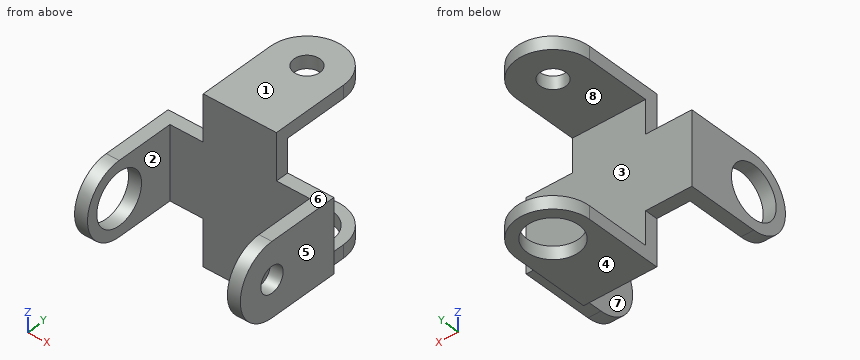
from build123d import *

# Parameters (mm, degrees)
BOSS_EXTRUDE1_DEPTH  = 5
SKETCH2_R            = 2.05
CUT_EXTRUDE1_DEPTH   = 5
SKETCH3_W            = 28.284271247
SKETCH3_H            = 5
BOSS_EXTRUDE3_DEPTH  = 5
SKETCH4_W            = 28.284271247
SKETCH4_H            = 5
BOSS_EXTRUDE4_DEPTH  = 54.01
BOSS_EXTRUDE5_DEPTH  = 5
SKETCH6_W            = 14.142135624
SKETCH6_H            = 14.14215
SKETCH6_W_2          = 12.862864377
SKETCH6_W_3          = 14.142135623
SKETCH6_W_4          = 12.862864376
BOSS_EXTRUDE7_DEPTH  = 5
SKETCH8_W            = 28.2843
SKETCH8_H            = 5
BOSS_EXTRUDE8_DEPTH  = 5
SKETCH10_W           = 5
SKETCH10_H           = 28.2843
BOSS_EXTRUDE9_DEPTH  = 22.6808
BOSS_EXTRUDE10_DEPTH = 5
SKETCH12_W           = 28.2843
SKETCH12_H           = 5
BOSS_EXTRUDE11_DEPTH = 5
BOSS_EXTRUDE12_START = -5
BOSS_EXTRUDE12_DEPTH = 5
SKETCH15_R           = 5
CUT_EXTRUDE3_DEPTH   = 5
SKETCH16_R           = 5
CUT_EXTRUDE4_DEPTH   = 14.1
SKETCH17_R           = 2.05
CUT_EXTRUDE5_DEPTH   = 8.1
SKETCH18_R           = 10
CUT_EXTRUDE6_DEPTH   = 5
SKETCH19_R           = 10
CUT_EXTRUDE7_DEPTH   = 5


with BuildPart() as part:
    # Model → Boss-Extrude1 (new body)
    with BuildSketch(Plane.XY):
        with BuildLine():
            Line((13.86155204, 4.132702322), (42.145823287, 4.132702322))
            Line((42.145823287, 4.132702322), (42.145823287, 29.132702322))
            ThreePointArc((42.145823287, 29.132702322), (28.003687664, 43.274837946), (13.86155204, 29.132702322))
            Line((13.86155204, 29.132702322), (13.86155204, 4.132702322))
        make_face()
    extrude(amount=BOSS_EXTRUDE1_DEPTH)

    # Sketch2 → Cut-Extrude1 (cut)
    with BuildSketch(Plane.XY.offset(5)):
        with Locations((28.003687664, 29.132702322)):
            Circle(SKETCH2_R)
    extrude(amount=-CUT_EXTRUDE1_DEPTH, mode=Mode.SUBTRACT)

    # Sketch3 → Boss-Extrude3 (add)
    with BuildSketch(Plane.XZ.offset(-4.132702322)):
        with Locations((28.003687664, 2.5)):
            Rectangle(SKETCH3_W, SKETCH3_H)
    extrude(amount=BOSS_EXTRUDE3_DEPTH)

    # Sketch4 → Boss-Extrude4 (add)
    with BuildSketch(Plane.XY.offset(5)):
        with Locations((28.003687664, 1.632702322)):
            Rectangle(SKETCH4_W, SKETCH4_H)
    extrude(amount=BOSS_EXTRUDE4_DEPTH)

    # Sketch5 → Boss-Extrude5 (add)
    with BuildSketch(Plane.XY.offset(59.01)):
        with BuildLine():
            Line((42.145823287, 4.132702322), (42.145823287, 29.132702322))
            ThreePointArc((42.145823287, 29.132702322), (28.003687664, 43.274837946), (13.86155204, 29.132702322))
            Line((13.86155204, 29.132702322), (13.86155204, 4.132702322))
            Line((13.86155204, 4.132702322), (13.86155204, -0.867297678))
            Line((13.86155204, -0.867297678), (42.145823287, -0.867297678))
            Line((42.145823287, -0.867297678), (42.145823287, 4.132702322))
        make_face()
    extrude(amount=BOSS_EXTRUDE5_DEPTH)

    # Sketch6 → Boss-Extrude7 (add)
    with BuildSketch(Plane.XZ.offset(0.867297678)):
        with Locations((20.932619852, 39.076075)):
            Rectangle(SKETCH6_W, SKETCH6_H)
        with Locations((48.577255476, 39.076075)):
            Rectangle(SKETCH6_W_2, SKETCH6_H)
        with Locations((35.074755476, 39.076075)):
            Rectangle(SKETCH6_W_3, SKETCH6_H)
        with Locations((7.430119852, 39.076075)):
            Rectangle(SKETCH6_W_4, SKETCH6_H)
        with Locations((7.430119852, 24.933925)):
            Rectangle(SKETCH6_W_4, SKETCH6_H)
        Polygon((28.003687664, 32.005), (13.86155204, 32.005), (13.86155204, 17.86285), (42.145823287, 17.86285), (42.145823287, 32.005), align=None)
        with Locations((48.577255476, 24.933925)):
            Rectangle(SKETCH6_W_2, SKETCH6_H)
    extrude(amount=-BOSS_EXTRUDE7_DEPTH)

    # Sketch8 → Boss-Extrude8 (add)
    with BuildSketch(Plane.ZY.offset(-0.998687664)):
        with Locations((32.005, 1.632702322)):
            Rectangle(SKETCH8_W, SKETCH8_H)
    extrude(amount=BOSS_EXTRUDE8_DEPTH)

    # Sketch10 → Boss-Extrude9 (add)
    with BuildSketch(Plane.XZ.offset(0.867297678)):
        with Locations((-1.501312336, 32.005)):
            Rectangle(SKETCH10_W, SKETCH10_H)
    extrude(amount=BOSS_EXTRUDE9_DEPTH)

    # Sketch11 → Boss-Extrude10 (add)
    with BuildSketch(Plane.ZY.offset(4.001312336)):
        with BuildLine():
            Line((46.14715, -23.548097678), (17.86285, -23.548097678))
            ThreePointArc((17.86285, -23.548097678), (32.005, -37.690247678), (46.14715, -23.548097678))
        make_face()
    extrude(amount=-BOSS_EXTRUDE10_DEPTH)

    # Sketch12 → Boss-Extrude11 (add)
    with BuildSketch(Plane(origin=(55.008687664, 0, 0), x_dir=(0, 0, -1), z_dir=(1, 0, 0))):
        with Locations((-32.005, 1.632702322)):
            Rectangle(SKETCH12_W, SKETCH12_H)
    extrude(amount=BOSS_EXTRUDE11_DEPTH)

    # Sketch14 → Boss-Extrude12 (add)
    with BuildSketch(Plane(origin=(60.008687664, 0, 0), x_dir=(0, 0, -1), z_dir=(1, 0, 0)).offset(BOSS_EXTRUDE12_START)):
        with BuildLine():
            Line((-17.86285, -0.867297678), (-46.14715, -0.867297678))
            Line((-46.14715, -0.867297678), (-46.14715, -23.548097678))
            ThreePointArc((-46.14715, -23.548097678), (-32.005, -37.690247678), (-17.86285, -23.548097678))
            Line((-17.86285, -23.548097678), (-17.86285, -0.867297678))
        make_face()
    extrude(amount=BOSS_EXTRUDE12_DEPTH)

    # Sketch15 → Cut-Extrude3 (cut)
    with BuildSketch(Plane.XY.offset(64.01)):
        with Locations((28.003687664, 29.132702322)):
            Circle(SKETCH15_R)
    extrude(amount=-CUT_EXTRUDE3_DEPTH, mode=Mode.SUBTRACT)

    # Sketch16 → Cut-Extrude4 (cut)
    with BuildSketch(Plane(origin=(60.008687664, 0, 0), x_dir=(0, 0, -1), z_dir=(1, 0, 0))):
        with Locations((-32.005, -23.548097678)):
            Circle(SKETCH16_R)
    extrude(amount=-CUT_EXTRUDE4_DEPTH, mode=Mode.SUBTRACT)

    # Sketch17 → Cut-Extrude5 (cut)
    with BuildSketch(Plane.ZY.offset(4.001312336)):
        with Locations(Location((32.005, -23.548097678, 0), (0, 0, 270))):
            Circle(SKETCH17_R)
    extrude(amount=-CUT_EXTRUDE5_DEPTH, mode=Mode.SUBTRACT)

    # Sketch18 → Cut-Extrude6 (cut)
    with BuildSketch(Plane(origin=(0, 0, 0), x_dir=(-1, 0, 0), z_dir=(0, 0, -1))):
        with Locations((-28.003687664, 29.132702322)):
            Circle(SKETCH18_R)
    extrude(amount=-CUT_EXTRUDE6_DEPTH, mode=Mode.SUBTRACT)

    # Sketch19 → Cut-Extrude7 (cut)
    with BuildSketch(Plane.ZY.offset(4.001312336)):
        with Locations(Location((32.005, -23.548097678, 0), (0, 0, 270))):
            Circle(SKETCH19_R)
    extrude(amount=-CUT_EXTRUDE7_DEPTH, mode=Mode.SUBTRACT)


solid = part.part
Work out the finished part from the listing and answer in its coordinate system (mm). Face numbers are marked on the shaded views. A direction names the side the tool comes from. Coordinates: 2 decimals unless noted, no trailing zeros. Write each loop counter-clockwise with the first axis right and the second up, starting at its lowest first coordinate (ties: lowest second). Pieces come first, ordered by that corner, then holes. Notation, with made-up numbers: M 42,33 L 95,33 A31 ccw 95,64 Z; hole C 80.5,70.5 d6. An arc over 180 degrees is marked long. Use one line per item in the form item = value. Start each with the question number.
1. Each of these flat-tipped pins is pushed along its axis until it touches: P1, Ø8, axis at x = 42.5, z = 41, coming from the +Y side; P2, Ø10, axis at x = 17.5, z = 28, coming from the -Y side; P3, Ø9, axis at x = 47, y = -6, coming from the -Z side; P4, Ø19.5, axis at y = 10, z = 5.5, coming from the +X side. Where does it stop, or does it pass through?
2. The part is cut by section B-B (x = 26.5). Give the vertices of the cut face in (y, z).
3. The part is cut by section C-C (y = 0.5). Give the vertices of the cut face in (x, z), plus the area to 3 significant figures.
4. A tool of negligible diameter and unlimited length cuts with its end or side. For the marked faces 4, 5, 6, 7 and 8, from which of +Z, -Z, +X, -X, +Y, -Y can it reach the whole face along a straight path? Write none if from no direction.
5. The part is cut by section A-A (y = 10.5). Give the vertices of the cut face in (x, z), plus the area to 3 significant figures.
6. The mould has two halves that part along Z. Classify the marked faces 1, 2 and 3: released by +Z, released by -Z, zero draft, split by the parting line, or undercut.
7. The part is cut by section D-D (z = 33). Give the vertices of the cut face in (x, y), plus the area to 3 significant figures.
8. Straight lines are drawn through the part: probe 1 along Z at (x, y) = (35.5, 38.5); probe 2 along X at (y, z) = (-15.5, 45); probe 3 along Y at (x, z) = (35, 36). For each, find the intervals that lie inside material, in ascending order. Write a range as from..to.
Evaluation:
q1.P1 = 4.13
q1.P2 = -0.87
q1.P3 = through
q1.P4 = 42.15
q2.outline = M -0.87,0 L 19.25,0 L 19.25,5 L 4.13,5 L 4.13,59.01 L 24.36,59.01 L 24.36,64.01 L -0.87,64.01 Z; M 33.9,59.01 L 43.19,59.01 L 43.19,64.01 L 33.9,64.01 Z; M 39.02,0 L 43.19,0 L 43.19,5 L 39.02,5 Z
q3.outline = M -4,17.86 L 13.86,17.86 L 13.86,0 L 42.15,0 L 42.15,17.86 L 60.01,17.86 L 60.01,46.15 L 42.15,46.15 L 42.15,64.01 L 13.86,64.01 L 13.86,46.15 L -4,46.15 Z
q3.area = 2,820 mm^2
q4.face_4 = -Z, +X, -X, +Y, -Y
q4.face_5 = +Z, -Z, +X, +Y, -Y
q4.face_6 = +Z, +X, +Y, -Y
q4.face_7 = +Z, -Z, -Y
q4.face_8 = +X, -X, +Y
q5.outline = M 13.86,0 L 42.15,0 L 42.15,5 L 13.86,5 Z; M 13.86,59.01 L 42.15,59.01 L 42.15,64.01 L 13.86,64.01 Z
q5.area = 283 mm^2
q6.face_1 = released by +Z
q6.face_2 = zero draft
q6.face_3 = undercut
q7.outline = M -4,-37.66 L 1,-37.66 L 1,-33.5 L -4,-33.5 Z; M -4,-13.6 L 1,-13.6 L 1,-0.87 L 55.01,-0.87 L 55.01,-18.65 L 60.01,-18.65 L 60.01,4.13 L -4,4.13 Z; M 55.01,-37.66 L 60.01,-37.66 L 60.01,-28.45 L 55.01,-28.45 Z
q7.area = 539 mm^2
q8.probe_1 = 0..5, 59.01..64.01
q8.probe_2 = -4..1, 55.01..60.01
q8.probe_3 = -0.87..4.13
